For this review, use the dimensioned drawing (mm, ordinates from the lowest corner) and the shaded views. A direction names the side the tool comes from. Round coordinates to 2 decimals unless told otherwise and drop trailing zeros. Loops run counter-clockwise (first coordinate to the right, second up) from the corner with the lowest first, then second, coordinate; pieces in that order, holes last. Notation, with made-up numbers: M -16,27 L -11,27 A19 ccw -11,36 Z; hole C -1,22.25 d11. An arc over 180 degrees is marked long. Answer as a JSON object with one key per item and string values. Group by question number.
Item 1: Consider section C-C (y = 46.5). Give the boundary of the cut face in (x, z), and give its area (3 significant figures).
Item 2: Consider section A-A (z = 36.65). Give the boundary of the cut face in (x, y).
Item 3: Tool access review of the marked faces 1, 2 and 3: name each direction out of +Z, -Z, +X, -X, +Y, -Y from which nothing blocks a thin tool from reaching the whole face with its end or side.
Item 4: Consider section B-B (x = 34.5). Give the boundary of the cut face in (y, z).
Item 5: Consider section D-D (x = 19). Give the boundary of the cut face in (y, z), and give its area (3 significant figures).
Item 6: Insertion check: P1, Ø12, axis at x = 49.5, y = 40.5, coming from the -Z side; P2, Ø5, axis at y = 36, z = 16, coming from the -X side; P3, Ø3.5, axis at x = 4.5, z = 36.65, coming from the +Y side; P4, Ø12, axis at y = 28, z = 18, coming from the +X side. Each pin has a flat end and moves straight along its axis. Give the tip position at first contact, or say it passes through.
Item 7: The part is to be moulded in two halves that separate along X. For the marked faces 4, 5, 6 and 7, say which applies: +X half, -X half, draft (parallel to the pull), parting line (faces both ways), or undercut.
Item 8: To check wall thickness, follow line 1 (Z direction, x = 50, y = 48.8); line 2 (X direction, y = 48.9, z = 36.65); line 3 (X direction, y = 19, z = 21.5). State the ranges of each line that lie inside material, in increasing order.
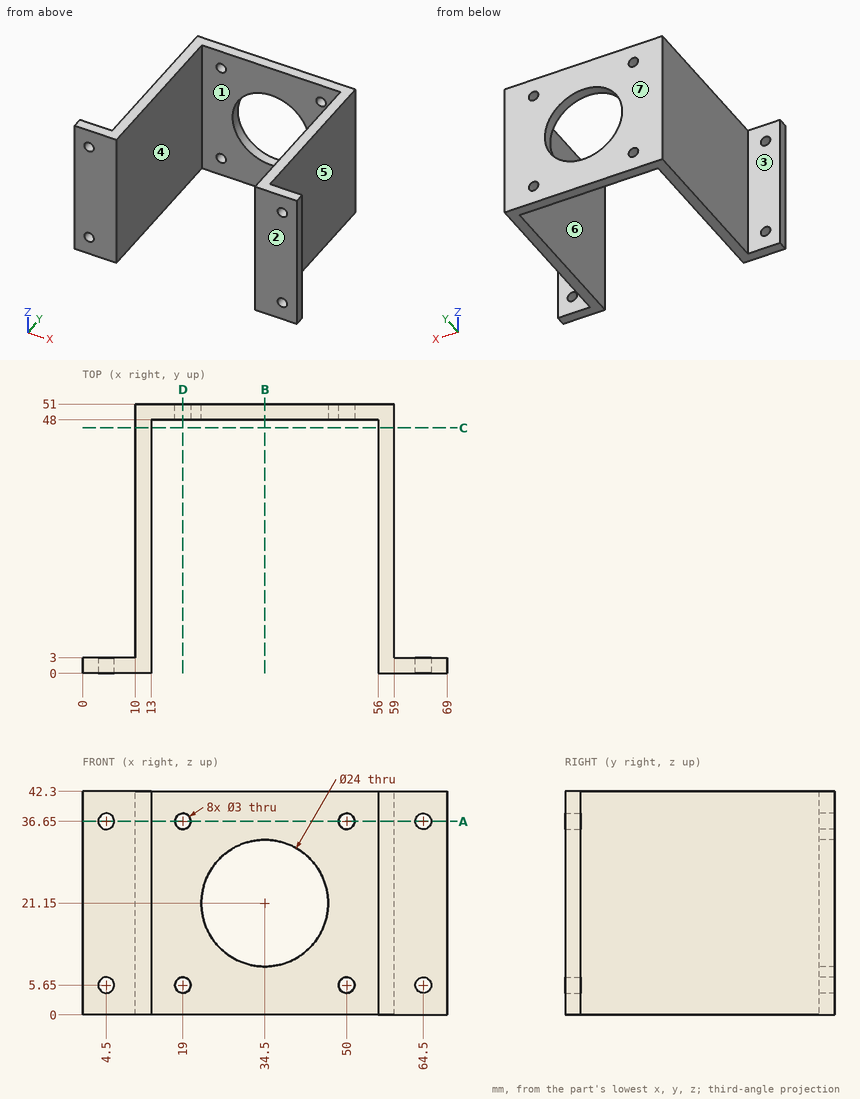
Geometry results:
{
 "1": {"outline": "M 10,0 L 13,0 L 13,42.3 L 10,42.3 Z; M 56,0 L 59,0 L 59,42.3 L 56,42.3 Z", "area": "254 mm^2"},
 "2": {"outline": "M 0,0 L 3,0 L 3,3 L 0,3 Z; M 6,0 L 13,0 L 13,48 L 17.5,48 L 17.5,51 L 10,51 L 10,3 L 6,3 Z; M 20.5,48 L 48.5,48 L 48.5,51 L 20.5,51 Z; M 51.5,48 L 56,48 L 56,0 L 63,0 L 63,3 L 59,3 L 59,51 L 51.5,51 Z; M 66,0 L 69,0 L 69,3 L 66,3 Z"},
 "3": {"face 1": "+Z, -Z, -Y", "face 2": "+Z, -Z, +X, -X, -Y", "face 3": "+Z, -Z, -X, +Y"},
 "4": {"outline": "M 48,0 L 51,0 L 51,9.15 L 48,9.15 Z; M 48,33.15 L 51,33.15 L 51,42.3 L 48,42.3 Z"},
 "5": {"outline": "M 48,0 L 51,0 L 51,4.15 L 48,4.15 Z; M 48,7.15 L 51,7.15 L 51,35.15 L 48,35.15 Z; M 48,38.15 L 51,38.15 L 51,42.3 L 48,42.3 Z", "area": "109 mm^2"},
 "6": {"P1": "passes through", "P2": "stops at x = 10", "P3": "stops at y = 3", "P4": "stops at x = 59"},
 "7": {"face 4": "undercut", "face 5": "+X half", "face 6": "undercut", "face 7": "draft"},
 "8": {"line 1": "z = 0 to 4.15, 7.15 to 35.15, 38.15 to 42.3", "line 2": "x = 10 to 17.5, 20.5 to 48.5, 51.5 to 59", "line 3": "x = 10 to 13, 56 to 59"}
}
